from build123d import *

# Parameters (mm, degrees)
BOSS_EXTRUDE1_DEPTH = 2


with BuildPart() as part:
    # Sketch2 → Boss-Extrude1 (new body)
    with BuildSketch(Plane(origin=(0, 0, 0), x_dir=(1, 0, 0), z_dir=(0, 1, 0))):
        with BuildLine():
            ThreePointArc((2.973213749, 0.4), (-2.121320344, 2.121320344), (-0.4, -2.973213749))
            Line((-0.4, -2.973213749), (-0.4, -2))
            Line((-0.4, -2), (0.4, -2))
            Line((0.4, -2), (0.4, -2.973213749))
            ThreePointArc((0.4, -2.973213749), (2.121320344, -2.121320344), (2.973213749, -0.4))
            Line((2.973213749, -0.4), (2, -0.4))
            Line((2, -0.4), (2, 0.4))
            Line((2, 0.4), (2.973213749, 0.4))
        make_face()
    extrude(amount=BOSS_EXTRUDE1_DEPTH)


solid = part.part
Geometry check sheet. Reference: the model listing, model coordinates, mm. A direction names the side the tool comes from. Coordinates: 2 decimals unless noted, no trailing zeros. Order: outer loops, then holes, each group sorted by start corner. A loop starts at its lowest first (then second) coordinate and runs counter-clockwise, first axis right, second up. Notation, with made-up numbers: (78, 85.25) - (93, 85.25) arc R32 ccw to (93, 116.25) - close; hole circle Ø3 at (61.5, 64). An arc over 180 degrees is marked (long way). One line per item, written item: value.
(1) Sectioned sample at D-D (x = 0). Enter the section's corners in (y, z), and give its area (3 significant figures).
Data:
outline: (0, -3) - (2, -3) - (2, 2) - (0, 2) - close
area: 10.0 mm^2
(2) Sectioned sample at B-B (x = 2.25). Enter the section's corners in (y, z), and give its area (3 significant figures).
Data:
outline: (0, -1.98) - (2, -1.98) - (2, -0.4) - (0, -0.4) - close; (0, 0.4) - (2, 0.4) - (2, 1.98) - (0, 1.98) - close
area: 6.34 mm^2
(3) Thickness scan on probe 1 along X at (y, z) = (0.3, 0.05); probe 2 along Z at (x, y) = (0.6, 1.15); probe 3 along Z at (x, y) = (2.25, 0.35). Record the ranges inside material, lowest first. Write a range as from..to.
Data:
probe 1: x = -3..2
probe 2: z = -2.94..2.94
probe 3: z = -1.98..-0.4, 0.4..1.98
(4) Depth check by flat-ended pin: pin 1 Ø0.5 at (y, z) = (0.5, 2.5) entering from +X; pin 2 Ø0.8 at (y, z) = (1.5, 2.5) entering from -X. Enter the tip coordinate at first touch or a pass-through.
Data:
pin 1: stops at x = 1.98
pin 2: stops at x = -2.14
(5) Access from +Z, -Z, +X, -X, +Y, -Y to the whole of each face (thin tool, end or side, straight path). Record for faces 4 (the face through (0, 2, 0)), 5 (the face through (0.4, 1, 2.5)), 6 (the face through (2.5, 1, -0.4)).
Data:
face 4: +Z, -Z, +X, -X, +Y
face 5: +Z, +Y, -Y
face 6: +X, +Y, -Y
(6) Release check for a two-part mould opening along X. For faces 1 (the face through (-0.4, 1, 2.5)), 2 (the face through (-2.05, 0.99, -2.19)), 3 (the face through (2.1, 0.99, 2.14)) record: +X half, -X half, draft (parallel to the pull), parting line (faces both ways), or undercut.
Data:
face 1: undercut
face 2: parting line
face 3: +X half
(7) Sectioned sample at C-C (z = 0). Enter the section's corners in (x, y), and give its area (3 significant figures).
Data:
outline: (-3, 0) - (2, 0) - (2, 2) - (-3, 2) - close
area: 10.0 mm^2
(8) Sectioned sample at A-A (y = 1). Enter the section's corners in (x, z), and give its area (3 significant figures).
Data:
outline: (-0.4, 2) - (-0.4, 2.97) arc R3 ccw (long way) to (2.97, -0.4) - (2, -0.4) - (2, 0.4) - (2.97, 0.4) arc R3 ccw to (0.4, 2.97) - (0.4, 2) - close
area: 26.7 mm^2
